Solid Edge part; units mm, degrees
sketch "Sketch1" plane through (0, 0, 0) normal (0, 0, 1) x (1, 0, 0)
  line L0 (-8, 26.3106) -> (-8, 22.096)
  arc A0 (-8, 22.096) -> (-0.9592, 23.4801) centre (0, 0) cw
  arc A1 (-0.9592, 23.4801) -> (0, 24.4792) centre (-1, 24.4792) ccw
  arc A2 (0, 24.4792) -> (0.9592, 23.4801) centre (1, 24.4792) ccw
  arc A3 (0.9592, 23.4801) -> (8, 22.096) centre (0, 0) cw
  line L1 (8, 22.096) -> (8, 26.3106)
  arc A4 (8, 26.3106) -> (3.319, 27.299) centre (0, 0) ccw
  arc A5 (3.319, 27.299) -> (2, 28.788) centre (3.5, 28.788) cw
  line L2 (2, 28.788) -> (2, 45.5)
  line L3 (2, 45.5) -> (0.2, 45.5)
  line L4 (0.2, 45.5) -> (0, 45.3)
  line L5 (0, 45.3) -> (-0.2, 45.5)
  line L6 (-0.2, 45.5) -> (-2, 45.5)
  line L7 (-2, 45.5) -> (-2, 28.788)
  arc A6 (-2, 28.788) -> (-3.319, 27.299) centre (-3.5, 28.788) cw
  arc A7 (-3.319, 27.299) -> (-8, 26.3106) centre (0, 0) ccw
revolve "RevolvedProtrusion1" add sketch "Sketch1" angle 360 about axis through (50, 0, 0) along (-1, 0, 0)
sketch "Sketch2" plane through (0, 0, 0) normal (1, 0, 0) x (0, 1, 0)
  line L0 (19.4672, -25.0182) -> (11.9328, -29.3682)
  line L1 (11.9328, -29.3682) -> (16.2828, -36.9026)
  line L2 (16.2828, -36.9026) -> (23.8172, -32.5526)
  line L3 (23.8172, -32.5526) -> (19.4672, -25.0182)
extrude "ExtrudedCutout_1" cut sketch "Sketch2" against normal blind 4 and the other way blind 4
sketch "Sketch3" plane through (0, 0, 0) normal (1, 0, 0) x (0, 1, 0)
  line L0 (-40.1, 4.35) -> (-40.1, -4.35)
  line L1 (-40.1, -4.35) -> (-31.4, -4.35)
  line L2 (-31.4, -4.35) -> (-31.4, 4.35)
  line L3 (-31.4, 4.35) -> (-40.1, 4.35)
extrude "ExtrudedCutout_2" cut sketch "Sketch3" against normal blind 4 and the other way blind 4
sketch "Sketch4" plane through (0, 0, 0) normal (1, 0, 0) x (0, 1, 0)
  line L0 (16.2828, 36.9026) -> (11.9328, 29.3682)
  line L1 (11.9328, 29.3682) -> (19.4672, 25.0182)
  line L2 (19.4672, 25.0182) -> (23.8172, 32.5526)
  line L3 (23.8172, 32.5526) -> (16.2828, 36.9026)
extrude "ExtrudedCutout_3" cut sketch "Sketch4" against normal blind 4 and the other way blind 4
properties material "Stainless steel"
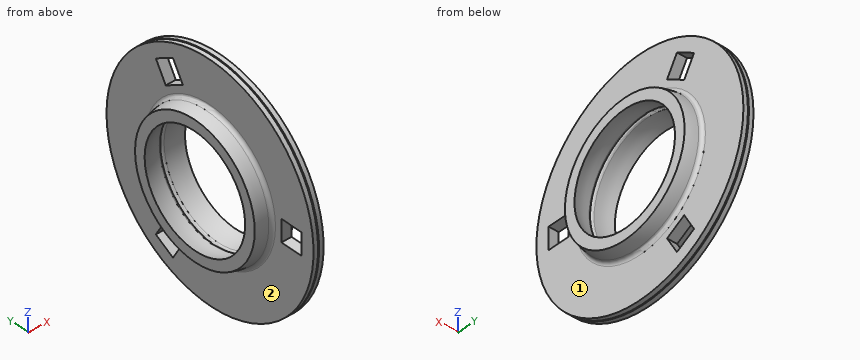
Source: CAD feature listing. Evaluate the final solid. Frame: model axes, mm. Face numbers are marked on the shaded views. A direction names the side the tool comes from. Round coordinates to 2 decimals unless told otherwise and drop trailing zeros. Order: outer loops, then holes, each group sorted by start corner. A loop starts at its lowest first (then second) coordinate and runs counter-clockwise, first axis right, second up. Notation, with made-up numbers: (34, 50) - (61, 50) arc R19 cw to (61, 69) - close; hole circle Ø5 at (42, -39). An arc over 180 degrees is marked (long way). Use a Markdown table: item, result. Add a question column.
1. Section query B-B (x = -6.25). Return the cut outline in (y, z).
2. First-contact query: pin 1 (2 mm diameter, centred on x = 1, z = -2, fed in from -Y); pin 2 (3 mm diameter, centred on x = -6, y = 17, fed in from +Z); pin 3 (12 mm diameter, centred on y = -15, z = 3.5, fed in from +X); pin 4 (1.2 mm diameter, centred on x = 0.5, z = -0.5, fed in from +Y). Flat tips, straight axial feed; report the tip coordinate or a pass-through.
3. Line query: probe 1 along X at (y, z) = (-6, -35); probe 2 along Y at (x, z) = (2.5, 16.5); probe 3 along Z at (x, y) = (1, 21). Output: solid intervals per line, ascending.
4. Section query C-C (z = 0). Give the number of separate pieces and of enclosed holes in the cut face, then the cut area to 3 significant figures.
5. Set-up query: the marked faces 1 and 2. Return all of +Z, -Z, +X, -X, +Y, -Y with unobstructed straight access to the full face (end or side cutting, diameter ignored); none if empty.
Derived:
| question | item | result |
|---|---|---|
| 1 | outline | circle Ø53.56 at (0, 0); hole circle Ø45.31 at (0, 0) |
| 2 | pin 1 | y = -45.49 |
| 2 | pin 2 | z = 21.98 |
| 2 | pin 3 | through |
| 2 | pin 4 | y = 45.5 |
| 3 | probe 1 | -2 to 2 |
| 3 | probe 2 | -22.21 to -16.54, 16.54 to 22.21 |
| 3 | probe 3 | -40.36 to -34.18, -27.67 to -10.5, 10.5 to 27.67, 34.18 to 40.36 |
| 4 | separate pieces | 3 |
| 4 | enclosed holes | 0 |
| 4 | area | 240 mm2 |
| 5 | face 1 | +X |
| 5 | face 2 | -X |
